Build history of the part. All positions in model axes, mm. Face numbers are marked on the shaded views. A direction names the side the tool comes from. Coordinates: 2 decimals unless noted, no trailing zeros. Loops run counter-clockwise (first coordinate to the right, second up) from the corner with the lowest first, then second, coordinate; pieces in that order, holes last.
Item 1: Drill centre lines: line 1 along Y through (x, z) = (0, 23.5); line 2 along Z through (x, y) = (1, 0.5); line 3 along Z through (x, y) = (-2, 2). Where is each one in solid material? Low to high.
Item 2: 3-axis set-ups, long thin cutter, end or side, ignore diameter. For the marked faces 1 and 2: which of +Z, -Z, +X, -X, +Y, -Y reach the whole face in a straight line?
Item 3: Cut at D-D (z = 8). List the corners of the cut face in (x, y), and give its area (3 significant figures).
Item 4: Flat gauge pins, fed straight in: pin 1 (2 mm diameter, centred on x = 0.5, z = -4, fed in from -Y); pin 2 (5 mm diameter, centred on x = 2, y = -4, fed in from -Z); pin 3 (3 mm diameter, centred on x = -4.5, y = 4.5, fed in from -Z). Where does each tip first touch, or does it go through?
Item 5: Cut at C-C (z = 22). List the corners of the cut face in (x, y).
from build123d import *

# Parameters (mm, degrees)
PAD_DEPTH    = 0.89
SKETCH001_R  = 5.59
PAD001_DEPTH = 24.89
SKETCH002_R  = 2.0828
PAD002_DEPTH = 14.25
SKETCH003_R  = 1.395
PAD003_DEPTH = 1
SKETCH004_R  = 0.76
PAD004_DEPTH = 3.18
SKETCH005_R  = 1.395
PAD005_DEPTH = 1
SKETCH006_R  = 2.11
POCKET_DEPTH = 10


with BuildPart() as part:
    # Sketch → Pad (new body)
    with BuildSketch(Plane.XY):
        with BuildLine():
            Line((-2.375952, 4.1275), (2.375952, 4.1275))
            ThreePointArc((-2.375952, 4.1275), (0, -4.7625), (2.375952, 4.1275))
        make_face()
    extrude(amount=PAD_DEPTH)

    # Sketch001 (on Face4 of Pad) → Pad001 (join)
    with BuildSketch(Plane.XY.offset(0.89)):
        Circle(SKETCH001_R)
    extrude(amount=PAD001_DEPTH)

    # Sketch002 (on Face6 of Pad001) → Pad002 (join)
    with BuildSketch(Plane(origin=(0, 0, 0), x_dir=(1, 0, 0), z_dir=(0, 0, -1))):
        Circle(SKETCH002_R)
    extrude(amount=PAD002_DEPTH)

    # Sketch003 (on Face8 of Pad002) → Pad003 (join)
    with BuildSketch(Plane(origin=(0, 0, -14.25), x_dir=(1, 0, 0), z_dir=(0, 0, -1))):
        Circle(SKETCH003_R)
    extrude(amount=PAD003_DEPTH)

    # Sketch004 (on Face10 of Pad003) → Pad004 (join)
    with BuildSketch(Plane(origin=(0, 0, -15.25), x_dir=(1, 0, 0), z_dir=(0, 0, -1))):
        Circle(SKETCH004_R)
    extrude(amount=PAD004_DEPTH)

    # Sketch005 (on Face12 of Pad004) → Pad005 (join)
    with BuildSketch(Plane(origin=(0, 0, -18.43), x_dir=(1, 0, 0), z_dir=(0, 0, -1))):
        Circle(SKETCH005_R)
    extrude(amount=PAD005_DEPTH)

    # Sketch006 (on Face14 of Pad005) → Pocket (cut)
    with BuildSketch(Plane.XY.offset(25.78)):
        Circle(SKETCH006_R)
    extrude(amount=-POCKET_DEPTH, mode=Mode.SUBTRACT)


solid = part.part
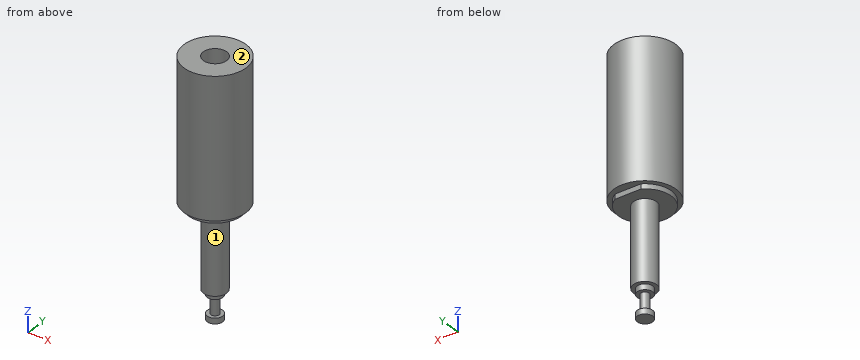
Filled sheet:
1. line 1: y = -5.59 to -2.11, 2.11 to 5.59
1. line 2: z = -19.43 to -18.43, -15.25 to 15.78
1. line 3: z = 0 to 25.78
2. face 1: -Z
2. face 2: +Z, +X, -X, +Y, -Y
3. outline: circle Ø11.18 at (0, 0)
3. area: 98.2 mm2
4. pin 1: stops at y = -2.08
4. pin 2: stops at z = -14.25
4. pin 3: stops at z = 0.89
5. outline: circle Ø11.18 at (0, 0); hole circle Ø4.22 at (0, 0)
